Here's how the part is built. I have some questions about the finished solid (model axes, mm). Give positions to 0.01 mm unless a question says otherwise; leave off trailing zeros. Write each loop counter-clockwise with the first axis right and the second up, starting at its lowest first coordinate (ties: lowest second). Pieces come first, ordered by that corner, then holes. Notation, with made-up numbers: (38.5, 20.25) - (85.5, 20.25) arc R32 cw to (85.5, 51.25) - close; hole circle Ø9 at (36, -8.75). An arc over 180 degrees is marked (long way). Write each question's results on one line, items separated by ' | '. Start each with the question number.
Item 1: Please list where these lines run through material, in increasing order: line 1 along Y through (x, z) = (40, 1.05); line 2 along X through (y, z) = (3.75, 1.7); line 3 along Y through (x, z) = (45, 0.6).
Item 2: Will this pin go through, and if not, where does the flat tip stop? P1, Ø3, axis at x = 10, y = 25, coming from the -Z side.
Item 3: Suppose I cut it at D-D on y = 25. List the corners of the cut face in (x, z) for me.
Item 4: Suppose I cut it at A-A on z = 1.55. List the corners of the cut face in (x, y) for me, then the cut area to 3 significant figures.
Item 5: Suppose I cut it at C-C on y = 9.5. List the corners of the cut face in (x, z) for me.
Item 6: Suppose I cut it at B-B on x = 10. List the corners of the cut face in (y, z) for me.
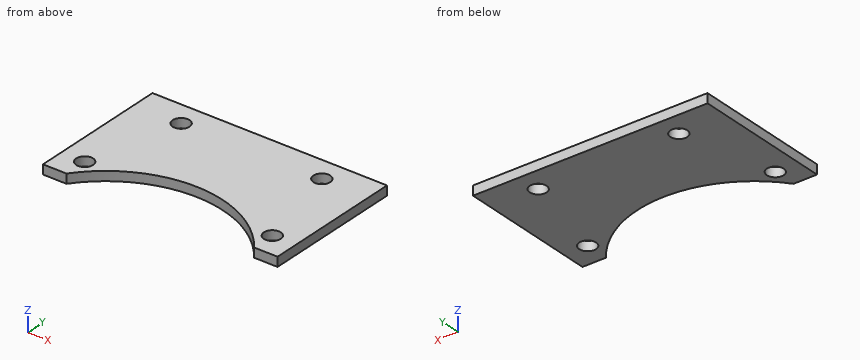
```python
from build123d import *

# Parameters (mm, degrees)
SKETCH_R  = 1.8
PAD_DEPTH = 2


with BuildPart() as part:
    # Sketch → Pad (new body)
    with BuildSketch(Plane.XY):
        with BuildLine():
            Line((5, 0), (0, 0))
            Line((0, 0), (0, 30))
            Line((0, 30), (50, 30))
            Line((50, 30), (50, 0))
            Line((50, 0), (45, 0))
            ThreePointArc((45, 0), (25, 10), (5, 0))
        make_face()
        with Locations((5, 5)):
            Circle(SKETCH_R, mode=Mode.SUBTRACT)
        with Locations((45, 5)):
            Circle(SKETCH_R, mode=Mode.SUBTRACT)
        with Locations((40, 25)):
            Circle(SKETCH_R, mode=Mode.SUBTRACT)
        with Locations((10, 25)):
            Circle(SKETCH_R, mode=Mode.SUBTRACT)
    extrude(amount=PAD_DEPTH)


solid = part.part
```
Checked values:
1) line 1: y = 5 to 23.2, 26.8 to 30 | line 2: x = 0 to 3.7, 6.3 to 8.46, 41.54 to 43.7, 46.3 to 50 | line 3: y = 0 to 3.2, 6.8 to 30
2) P1: passes through
3) outline: (0, 0) - (8.2, 0) - (8.2, 2) - (0, 2) - close; (11.8, 0) - (38.2, 0) - (38.2, 2) - (11.8, 2) - close; (41.8, 0) - (50, 0) - (50, 2) - (41.8, 2) - close
4) outline: (0, 0) - (5, 0) arc R25 cw to (45, 0) - (50, 0) - (50, 30) - (0, 30) - close; hole circle Ø3.6 at (5, 5); hole circle Ø3.6 at (10, 25); hole circle Ø3.6 at (40, 25); hole circle Ø3.6 at (45, 5) | area: 1,180 mm^2
5) outline: (0, 0) - (20.03, 0) - (20.03, 2) - (0, 2) - close; (29.97, 0) - (50, 0) - (50, 2) - (29.97, 2) - close
6) outline: (5, 0) - (23.2, 0) - (23.2, 2) - (5, 2) - close; (26.8, 0) - (30, 0) - (30, 2) - (26.8, 2) - close
